The model under review builds one solid part; all positions refer to its coordinate system, in mm. A direction names the side the tool comes from. Round coordinates to 2 decimals unless told otherwise and drop trailing zeros. Write each loop counter-clockwise with the first axis right and the second up, starting at its lowest first coordinate (ties: lowest second). Pieces come first, ordered by that corner, then holes. Notation, with made-up numbers: (-21.75, 5.5) - (-4.75, 5.5) arc R25 cw to (-4.75, 25.5) - close; hole circle Ø2 at (48.25, 8). An arc over 180 degrees is marked (long way). Use one line per item in the form item = value.
from build123d import *
from build123d.topology import SkipClean

# Parameters (mm, degrees)
BOSS_EXTRUDE1_DEPTH            = 46.6
CUT_EXTRUDE1_REACH             = 137.409
SKETCH2_R                      = 19
SKETCH3_W                      = 3
SKETCH3_H                      = 30.7
BOSS_EXTRUDE2_DEPTH            = 120
SKETCH4_W                      = 5
SKETCH4_H                      = 7.85
BOSS_EXTRUDE3_DEPTH            = 120
SKETCH6_W                      = 3
SKETCH6_H                      = 35.7
BOSS_EXTRUDE4_DEPTH            = 120
SKETCH8_W                      = 4.95
SKETCH8_H                      = 35.7
BOSS_EXTRUDE5_DEPTH            = 120
BOSS_EXTRUDE7_DEPTH            = 117
CHAMFER2_SIZE                  = 8
M3_CLEARANCE_HOLE1_D           = 3.4
M3_CLEARANCE_HOLE1_ON_FACE_2_D = 3.4
SKETCH12_W                     = 8
SKETCH12_H                     = 17.7
CUT_EXTRUDE4_DEPTH             = 140.841195647
CHAMFER4_SIZE                  = 4
CHAMFER5_SIZE                  = 2
CUT_EXTRUDE5_START             = 6.3
CUT_EXTRUDE5_DEPTH             = 35.7
CUT_EXTRUDE6_START             = -70
CUT_EXTRUDE6_DEPTH             = 61.400086431
CUT_EXTRUDE7_START             = -4.5
CUT_EXTRUDE7_DEPTH             = 6.7
M3_CLEARANCE_HOLE2_D           = 3.6
M3_CLEARANCE_HOLE2_DEPTH       = 12.65
CHAMFER6_SIZE                  = 2.2
CUT_EXTRUDE8_DEPTH             = 131.400086431


# Read off the part's stored shape, not the designer's step: Cut-Extrude5
with BuildPart() as part:
    # Sketch1 → Boss-Extrude1 (new body)
    with BuildSketch(Plane.XY):
        Polygon((0, 0), (0, 42), (-120, 42), (-120, 37), (-3, 37), (-3, 9.3), (-18, 9.3), (-18, 6.3), (-10, 6.3), (-10, 0), align=None)
    extrude(amount=BOSS_EXTRUDE1_DEPTH)

    # Sketch2 → Cut-Extrude1 (cut, up to next)
    with BuildSketch(Plane(origin=(0, 0, 0), x_dir=(0, 0, -1), z_dir=(1, 0, 0)), mode=Mode.PRIVATE) as cut_extrude1_sk1:
        with Locations((-23.3, 20)):
            Circle(SKETCH2_R)
    cut_extrude1_tool1 = extrude(cut_extrude1_sk1.sketch, amount=-CUT_EXTRUDE1_REACH, mode=Mode.PRIVATE) & part.part
    add(cut_extrude1_tool1.solids().sort_by_distance((0, 20, 23.3))[0], mode=Mode.SUBTRACT)

    # Sketch3 → Boss-Extrude2 (add)
    with BuildSketch(Plane.ZY.offset(3)):
        with Locations((45.1, 21.65)):
            Rectangle(SKETCH3_W, SKETCH3_H)
    extrude(amount=BOSS_EXTRUDE2_DEPTH)

    # Sketch4 → Boss-Extrude3 (add)
    with BuildSketch(Plane(origin=(0, 0, 0), x_dir=(0, 0, -1), z_dir=(1, 0, 0))):
        with Locations((-49.1, 10.225)):
            Rectangle(SKETCH4_W, SKETCH4_H)
    extrude(amount=-BOSS_EXTRUDE3_DEPTH)

    # Sketch6 → Boss-Extrude4 (add)
    with BuildSketch(Plane(origin=(0, 0, 0), x_dir=(0, 0, -1), z_dir=(1, 0, 0))):
        with Locations((-1.5, 24.15)):
            Rectangle(SKETCH6_W, SKETCH6_H)
    extrude(amount=-BOSS_EXTRUDE4_DEPTH)

    # Sketch8 → Boss-Extrude5 (add)
    with BuildSketch(Plane(origin=(0, 0, 0), x_dir=(0, 0, -1), z_dir=(1, 0, 0))):
        with Locations((2.475, 24.15)):
            Rectangle(SKETCH8_W, SKETCH8_H)
    extrude(amount=-BOSS_EXTRUDE5_DEPTH)

    # Sketch14 → Boss-Extrude7 (add)
    with SkipClean():  # the faces are left unmerged after this step: merging them gives an invalid solid
        with BuildSketch(Plane.ZY.offset(3)):
            with BuildLine():
                Line((6.365553185, 28.615364824), (3, 22))
                Line((3, 22), (3, 37))
                Line((3, 37), (14.814718626, 37))
                ThreePointArc((14.814718626, 37), (9.91657099, 33.486431253), (6.365553185, 28.615364824))
            make_face()
            with BuildLine():
                Line((40.234446815, 28.615364824), (43.6, 22))
                Line((43.6, 22), (43.6, 37))
                Line((43.6, 37), (31.785281374, 37))
                ThreePointArc((31.785281374, 37), (36.68342901, 33.486431253), (40.234446815, 28.615364824))
            make_face()
        extrude(amount=BOSS_EXTRUDE7_DEPTH)

    # Chamfer2
    chamfer2_edges = [part.edges().sort_by_distance(p)[0] for p in [
        (0, 24.15, -4.95),
    ]]
    chamfer(chamfer2_edges, length=CHAMFER2_SIZE)

    # M3 Clearance Hole1 (through all)
    with Locations(Plane(origin=(-14, 0, -0.95), x_dir=(0, 0, -1), z_dir=(0, -1, 0))):
        with Locations((0, 0)):
            Hole(M3_CLEARANCE_HOLE1_D / 2)

    # M3 Clearance Hole1 on face 2 (through all)
    with Locations(Plane(origin=(-78.5, -3, -0.95), x_dir=(0, 0, -1), z_dir=(0, -1, 0))):
        with Locations((0, 0)):
            Hole(M3_CLEARANCE_HOLE1_ON_FACE_2_D / 2)

    # Sketch12 → Cut-Extrude4 (cut, through all)
    with SkipClean():  # the faces are left unmerged after this step: merging them gives an invalid solid
        with BuildSketch(Plane(origin=(0, 0, 0), x_dir=(0, 0, -1), z_dir=(1, 0, 0))):
            with Locations((0.95, 33.15)):
                Rectangle(SKETCH12_W, SKETCH12_H)
        extrude(amount=-CUT_EXTRUDE4_DEPTH, mode=Mode.SUBTRACT)

    # Chamfer4
    chamfer4_edges = [part.edges().sort_by_distance(p)[0] for p in [
        (-60, 42, 3.05),
    ]]
    chamfer(chamfer4_edges, length=CHAMFER4_SIZE)

    # Chamfer5
    chamfer5_edges = [part.edges().sort_by_distance(p)[0] for p in [
        (-60, 24.3, 3.05),
    ]]
    chamfer(chamfer5_edges, length=CHAMFER5_SIZE)

    # Cut-Extrude5 outline → Cut-Extrude5 (cut)
    with SkipClean():  # the faces are left unmerged after this step: merging them gives an invalid solid
        with BuildSketch(Plane(origin=(0, 0, 0), x_dir=(1, 0, 0), z_dir=(0, 1, 0)).offset(CUT_EXTRUDE5_START)):
            with BuildLine():
                Line((-120, -51.6), (-105.764031959, -51.6))
                ThreePointArc((-105.764031959, -51.6), (-112.149994188, -23.327677022), (-105.787782122, 4.95))
                Line((-105.787782122, 4.95), (-120, 4.95))
                Line((-120, 4.95), (-120, -43.6))
                Line((-120, -43.6), (-123, -43.6))
                Line((-123, -43.6), (-123, -46.6))
                Line((-123, -46.6), (-120, -46.6))
                Line((-120, -46.6), (-120, -51.6))
            make_face()
        extrude(amount=CUT_EXTRUDE5_DEPTH, mode=Mode.SUBTRACT)

    # Sketch16 → Cut-Extrude6 (cut, through all)
    with SkipClean():  # the faces are left unmerged after this step: merging them gives an invalid solid
        with BuildSketch(Plane(origin=(0, 0, 0), x_dir=(0, 0, -1), z_dir=(1, 0, 0)).offset(CUT_EXTRUDE6_START)):
            with BuildLine():
                Line((-3.05, 26.3), (-3.05, 42))
                Line((-3.05, 42), (-23.3, 42))
                Line((-23.3, 42), (-17.040626863, 40.045454545))
                ThreePointArc((-17.040626863, 40.045454545), (-9.51709951, 35.84397848), (-4.314345847, 28.97468308))
                Line((-4.314345847, 28.97468308), (-3.05, 26.3))
            make_face()
        extrude(amount=-CUT_EXTRUDE6_DEPTH, mode=Mode.SUBTRACT)

    # Sketch18 → Cut-Extrude7 (cut)
    with SkipClean():  # the faces are left unmerged after this step: merging them gives an invalid solid
        with BuildSketch(Plane(origin=(0, 14.15, 0), x_dir=(1, 0, 0), z_dir=(0, 1, 0)).offset(CUT_EXTRUDE7_START)):
            Polygon((-10.593633412, -47.55), (-12.296816706, -44.6), (-15.703183294, -44.6), (-17.406366588, -47.55), (-15.703183294, -50.5), (-12.296816706, -50.5), align=None)
            Polygon((-81.906366588, -47.55), (-80.203183294, -50.5), (-76.796816706, -50.5), (-75.093633412, -47.55), (-76.796816706, -44.6), (-80.203183294, -44.6), align=None)
        extrude(amount=CUT_EXTRUDE7_DEPTH, mode=Mode.SUBTRACT)

    # M3 Clearance Hole2
    with Locations(Plane(origin=(-78.5, -3, 47.55), x_dir=(0, 0, -1), z_dir=(0, -1, 0))):
        with Locations((0, 0), (0, 64.5)):
            Hole(M3_CLEARANCE_HOLE2_D / 2, depth=M3_CLEARANCE_HOLE2_DEPTH)

    # Chamfer6
    chamfer6_edges = [part.edges().sort_by_distance(p)[0] for p in [
        (-94.625687487, 14.15, 46.6),
        (-46.25, 14.15, 46.6),
        (-5.571058084, 14.15, 46.6),
    ]]
    chamfer(chamfer6_edges, length=CHAMFER6_SIZE)

    # Sketch23 → Cut-Extrude8 (cut, through all)
    with SkipClean():  # the faces are left unmerged after this step: merging them gives an invalid solid
        with BuildSketch(Plane(origin=(0, 0, 0), x_dir=(0, 0, -1), z_dir=(1, 0, 0))):
            Polygon((-48.8, 14.15), (-51.6, 11.35), (-51.6, 14.15), align=None)
        extrude(amount=-CUT_EXTRUDE8_DEPTH, mode=Mode.SUBTRACT)


solid = part.part
(1) Add section C-C on x = -48. Write out the cut boundary in (y, z), then the cut area to 3 significant figures.
Geometry results:
outline = (6.3, -4.95) - (24.3, -4.95) - (24.3, 1.05) - (26.3, 3.05) - (38, 3.05) - (42, 7.05) - (42, 46.6) - (16.35, 46.6) - (11.35, 51.6) - (6.3, 51.6) - (6.3, 43.6) - (22, 43.6) - (28.62, 40.23) arc R19 cw to (28.62, 6.37) - (22, 3) - (6.3, 3) - close
area = 595 mm2
(2) Machinability: for faces 5 (the flat face through (-18, 8, 6)), 6 (the flat face through (-90.78, 41.036, 20.214)), 7 (the flat face through (-35, 32, 3.05)), which of the approach directions +Z, -Z, +X, -X, +Y, -Y give a long, thin tool a straight path to every point of the face, cutting with its end or side? Answer none if there is none.
Geometry results:
face_5 = -X, -Y
face_6 = -Z, -X, +Y
face_7 = -Z, +X, -X, +Y
(3) Add section A-A on y = 20. Write out the cut boundary in (x, z).
Geometry results:
outline = (-108.95, 3) arc R65.9 ccw to (-105.79, -4.95) - (-8, -4.95) - (0, 3.05) - (0, 4.3) - (-3, 4.3) - (-3, 3) - close; (-108.95, 43.6) - (-3, 43.6) - (-3, 42.3) - (0, 42.3) - (0, 46.6) - (-107.89, 46.6) arc R65.9 ccw to start; hole circle Ø3.4 at (-78.5, -0.95); hole circle Ø3.4 at (-14, -0.95)
(4) Add section B-B on x = -78.5. Count the separate pieces of the cut face and the enclosed holes in it, then the cut area to 3 significant figures.
Geometry results:
separate_pieces = 3
enclosed_holes = 0
area = 399 mm2
(5) The part is to be moulded in two halves that separate along X. For faces 1 (the flat face through (-75.93, 12.95, 46.1)), 2 (the flat face through (-54, 6.3, 48)), 3 (the cylindrical face through (-13.93, 15.43, -2.65)), 4 (the flat face through (-18, 8, 41)), say which applies: +X half, -X half, draft (parallel to the pull), parting line (faces both ways), or undercut.
Geometry results:
face_1 = undercut
face_2 = draft
face_3 = undercut
face_4 = -X half
(6) To check wall thickness, follow L1, parallel to Z at x = -78.5, y = 14.75; L2, parallel to X at y = 10, z = 0; L3, parallel to Z at x = -99, y = 21. State the ranges of each line that lie inside material, in increasing order.
Geometry results:
L1 = -4.95 to -2.65, 0.75 to 3, 43.6 to 44.6
L2 = -107.89 to -79.91, -77.09 to -15.41, -12.59 to -3.05
L3 = -4.95 to 3, 43.6 to 46.6
(7) Insertion check: P1, Ø10, axis at x = -27.5, y = 37, coming from the -Z side; P2, Ø1.6, axis at x = -78, z = 46, coming from the -Y side; P3, Ø3, axis at x = -38.5, z = -2.5, coming from the +Y side. Each pin has a flat end and moves straight along its axis. Give the tip position at first contact, or say it passes through.
Geometry results:
P1 = 3.05
P2 = 6.3
P3 = 24.3
